Design review of the part shown in the three views and the two pictorial views. Dimensions are in mm from the part's minimum x, y and z. Give positions to 0.01 mm unless a question says otherwise; leave off trailing zeros. Order: outer loops, then holes, each group sorted by start corner. A loop starts at its lowest first (then second) coordinate and runs counter-clockwise, first axis right, second up. Notation, with made-up numbers: M 21,-5 L 45,-5 A32 ccw 45,34 Z; hole C 74.25,66.5 d11. An arc over 180 degrees is marked long. Answer as a JSON object with one key per item and string values.
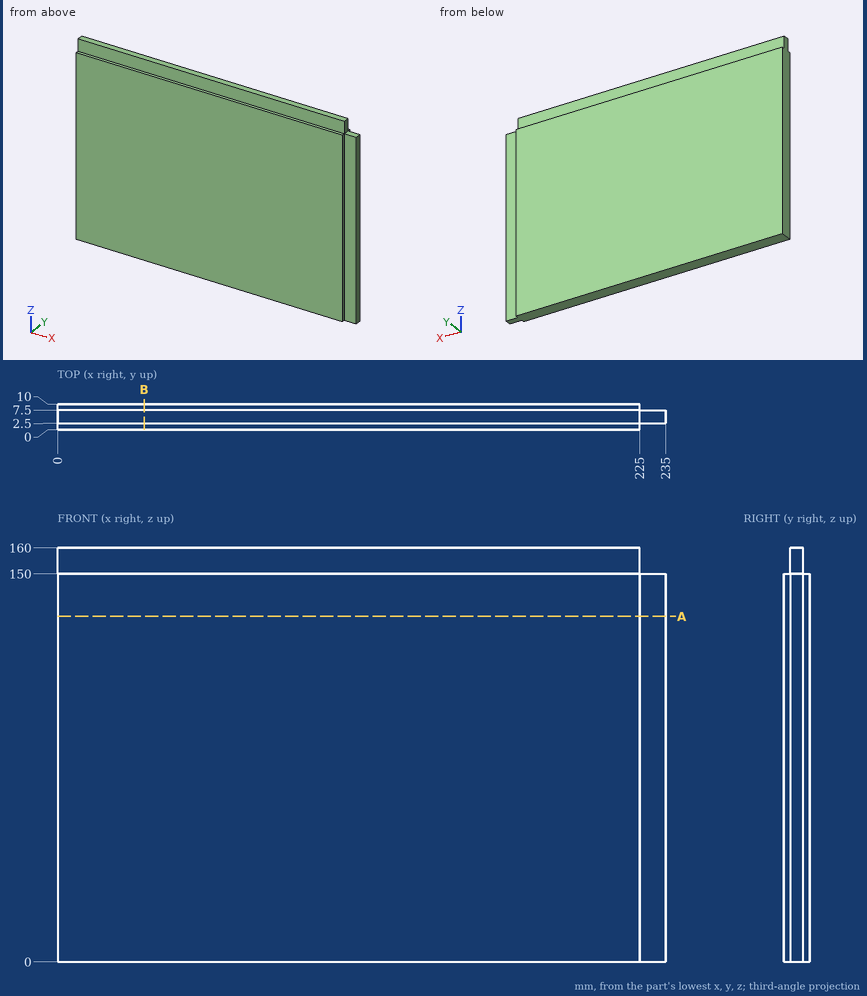
(1) Insertion check: pin 1 (5 mm diameter, centred on x = 83, z = 154.5, fed in from +Y); pin 2 (8 mm diameter, centred on x = 231, z = 100.5, fed in from -Y); pin 3 (2.5 mm diameter, centred on x = 228.5, y = 5, fed in from +Z). Each pin has a flat end and moves straight along its axis. Give the tip position at first contact, or say it passes through.
Checked values:
{"pin 1": "stops at y = 7.5", "pin 2": "stops at y = 2.5", "pin 3": "stops at z = 150"}
(2) We need section A-A (z = 133.5). Write out the cut boundary in (x, y).
Checked values:
{"outline": "M 0,0 L 225,0 L 225,2.5 L 235,2.5 L 235,7.5 L 225,7.5 L 225,10 L 0,10 Z"}
(3) We need section B-B (x = 33.5). Write out the cut boundary in (y, z).
Checked values:
{"outline": "M 0,0 L 10,0 L 10,150 L 7.5,150 L 7.5,160 L 2.5,160 L 2.5,150 L 0,150 Z"}
(4) To check wall thickness, follow L1, parallel to Y at x = 123, z = 150.5; L2, parallel to X at y = 8.75, z = 143.5; L3, parallel to Z at x = 220.5, y = 9.75. State the ranges of each line that lie inside material, in increasing order. Write a range as from..to.
Checked values:
{"L1": "y = 2.5..7.5", "L2": "x = 0..225", "L3": "z = 0..150"}
